The listing builds one solid part. Answer for the finished solid, in the listing's coordinates (mm). Face numbers are marked on the shaded views. A direction names the side the tool comes from. Coordinates: 2 decimals unless noted, no trailing zeros. Loops run counter-clockwise (first coordinate to the right, second up) from the corner with the lowest first, then second, coordinate; pieces in that order, holes last. Notation, with made-up numbers: (31.5, 53.5) -> (54.5, 53.5) arc R6 ccw to (54.5, 61.5) -> close; hole circle Ø3 at (73.5, 60). An arc over 180 degrees is marked (long way). Answer in a Markdown table with one row per item.
```python
from build123d import *

# Parameters (mm, degrees)
SKETCH1_R           = 25.4
BOSS_EXTRUDE2_DEPTH = 6.35
SKETCH2_R           = 19.05
BOSS_EXTRUDE3_DEPTH = 25.4
SKETCH3_R           = 6.35
CUT_EXTRUDE2_DEPTH  = 48.941448664


with BuildPart() as part:
    # Sketch1 → Boss-Extrude2 (new body)
    with BuildSketch(Plane.XY):
        Circle(SKETCH1_R)
    extrude(amount=-BOSS_EXTRUDE2_DEPTH)

    # Sketch2 → Boss-Extrude3 (add)
    with BuildSketch(Plane(origin=(0, 0, -6.35), x_dir=(-1, 0, 0), z_dir=(0, 0, -1))):
        Circle(SKETCH2_R)
    extrude(amount=BOSS_EXTRUDE3_DEPTH)

    # Sketch3 → Cut-Extrude2 (cut, through all)
    with BuildSketch(Plane.XY):
        Circle(SKETCH3_R)
    extrude(amount=-CUT_EXTRUDE2_DEPTH, mode=Mode.SUBTRACT)


solid = part.part
```
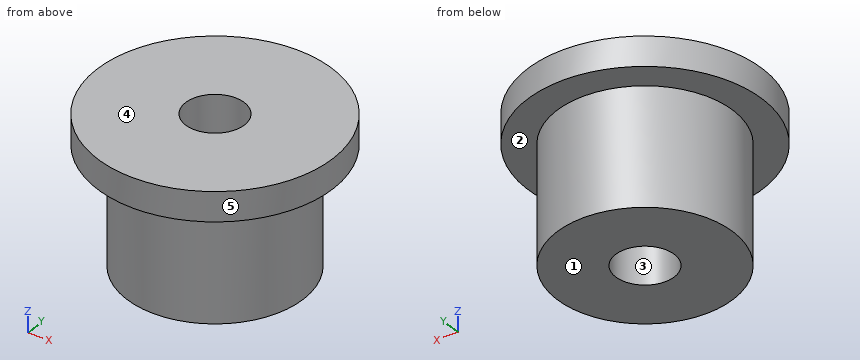
Item 1: A tool of negligible diameter and unlimited length cuts with its end or side. For the marked faces 1 and 2, from which of +Z, -Z, +X, -X, +Y, -Y can it reach the whole face along a straight path? Write none if from no direction.
Findings below:
| item | result |
|---|---|
| face 1 | -Z, +X, -X, +Y, -Y |
| face 2 | -Z |
Item 2: Determine the mould class of the marked faces 3, 4 and 5 for opening direction Y: +Y half, -Y half, draft (parallel to the pull), parting line (faces both ways), or undercut.
Findings below:
| item | result |
|---|---|
| face 3 | undercut |
| face 4 | draft |
| face 5 | parting line |
Item 3: A cutting plane is placed at A-A, the plane y = 0. Determine the outline of the cut face in (x, z), plus the area to 3 significant figures.
Findings below:
| item | result |
|---|---|
| outline | (-25.4, -6.35) -> (-19.05, -6.35) -> (-19.05, -31.75) -> (-6.35, -31.75) -> (-6.35, 0) -> (-25.4, 0) -> close; (6.35, -31.75) -> (19.05, -31.75) -> (19.05, -6.35) -> (25.4, -6.35) -> (25.4, 0) -> (6.35, 0) -> close |
| area | 887 mm2 |
Item 4: A cutting plane is placed at D-D, the plane y = 8. Determine the outline of the cut face in (x, z), plus the area to 3 significant figures.
Findings below:
| item | result |
|---|---|
| outline | (-24.11, -6.35) -> (-17.29, -6.35) -> (-17.29, -31.75) -> (17.29, -31.75) -> (17.29, -6.35) -> (24.11, -6.35) -> (24.11, 0) -> (-24.11, 0) -> close |
| area | 1,180 mm2 |
Item 5: Flat-ended cylindrical pins translate along their axes: pin 1 Ø8 at (x, z) = (12.5, -22.5) entering from +Y; pin 2 Ø1.5 at (y, z) = (15.5, -20) entering from -X; pin 3 Ø5 at (x, z) = (-19.5, -7) entering from -Y. Find the tip coordinate at first contact, or state that the pin passes through.
Findings below:
| item | result |
|---|---|
| pin 1 | stops at y = 17.05 |
| pin 2 | stops at x = -12.06 |
| pin 3 | stops at y = -18.79 |
Item 6: Find the intervals of material crossed by probe 1 along Y at (x, z) = (0, -24); probe 2 along Z at (x, y) = (17, -11); probe 3 along X at (y, z) = (1, -29), in increasing order.
Findings below:
| item | result |
|---|---|
| probe 1 | y = -19.05 to -6.35, 6.35 to 19.05 |
| probe 2 | z = -6.35 to 0 |
| probe 3 | x = -19.02 to -6.27, 6.27 to 19.02 |
Item 7: A cutting plane is placed at C-C, the plane z = -4.5. Determine the outline of the cut face in (x, y).
Findings below:
| item | result |
|---|---|
| outline | circle Ø50.8 at (0, 0); hole circle Ø12.7 at (0, 0) |
